For this review, use the dimensioned drawing (mm, ordinates from the lowest corner) and the shaded views. Give positions to 0.01 mm unless a question says otherwise; leave off trailing zeros. Write each loop counter-clockwise with the first axis right and the second up, starting at its lowest first coordinate (ties: lowest second). Pieces come first, ordered by that corner, then holes.
1) For P1, Ø1.5, axis at y = 90, z = 3.5, coming from the -X side; P2, Ø1.3, axis at y = 2.5, z = 2, coming from the +X side; P3, Ø1.5, axis at x = 128.5, z = 1, coming from the -Y side, all flat-tipped, find the tip position at first contact; note any pin that passes through.
2) We need section B-B on y = 32.5. Give the boundary of the cut face in (x, z).
3) We need section C-C on x = 22. Give the boundary of the cut face in (y, z), and give its area (4 significant figures).
4) Wall thickness on line 1 along Y through (x, z) = (136, 3.4); line 2 along X through (y, z) = (114, 1.9); line 3 along X through (y, z) = (51, 1): over which ranges is each line inside the solid? List them lowest first.
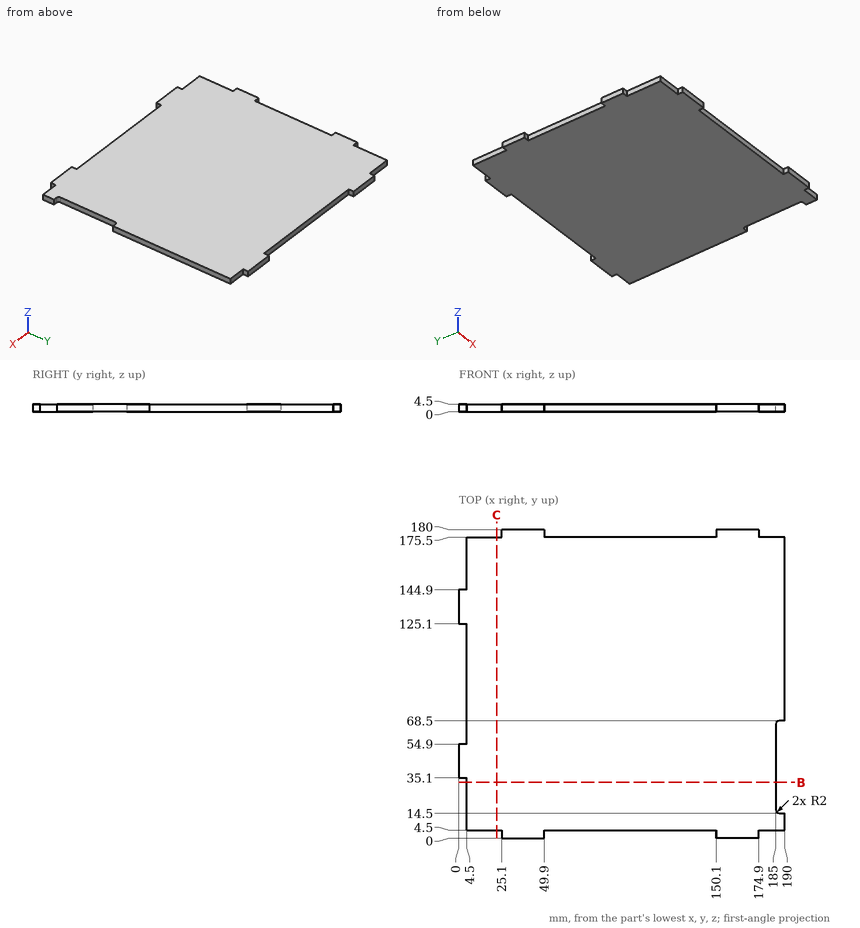
Results list:
1. P1: stops at x = 4.5
1. P2: stops at x = 174.9
1. P3: stops at y = 4.5
2. outline: (4.5, 0) - (185, 0) - (185, 4.5) - (4.5, 4.5) - close
3. outline: (4.5, 0) - (175.5, 0) - (175.5, 4.5) - (4.5, 4.5) - close
3. area: 769.5 mm2
4. line 1: y = 4.5 to 175.5
4. line 2: x = 4.5 to 190
4. line 3: x = 0 to 185
